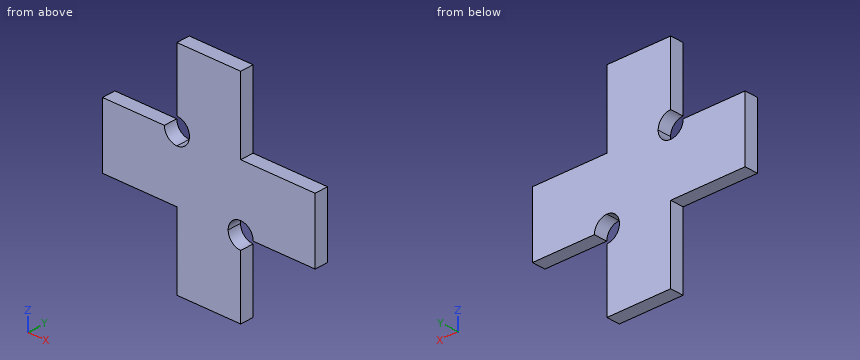
```python
from build123d import *

# Parameters (mm, degrees)
BOSS_EXTRUDE1_DEPTH = 1.6


with BuildPart() as part:
    # Sketch1 → Boss-Extrude1 (new body)
    with BuildSketch(Plane(origin=(0, 0, 0), x_dir=(1, 0, 0), z_dir=(0, 1, 0))):
        with BuildLine():
            Line((-12.7, -3.81), (-5.31, -3.81))
            ThreePointArc((-5.31, -3.81), (-4.870660172, -2.749339828), (-3.81, -2.31))
            Line((-3.81, -2.31), (-3.81, 3.81))
            Line((-3.81, 3.81), (-12.7, 3.81))
            Line((-12.7, 3.81), (-12.7, -3.81))
        make_face()
        with BuildLine():
            Line((-2.31, -3.81), (3.81, -3.81))
            Line((3.81, -3.81), (3.81, 2.31))
            ThreePointArc((3.81, 2.31), (2.749339828, 2.749339828), (2.31, 3.81))
            Line((2.31, 3.81), (-3.81, 3.81))
            Line((-3.81, 3.81), (-3.81, -2.31))
            ThreePointArc((-3.81, -2.31), (-2.749339828, -2.749339828), (-2.31, -3.81))
        make_face()
        with BuildLine():
            Line((-3.81, -12.7), (3.81, -12.7))
            Line((3.81, -12.7), (3.81, -3.81))
            Line((3.81, -3.81), (-2.31, -3.81))
            ThreePointArc((-2.31, -3.81), (-2.749339828, -4.870660172), (-3.81, -5.31))
            Line((-3.81, -5.31), (-3.81, -12.7))
        make_face()
        with BuildLine():
            Line((3.81, 2.31), (3.81, -3.81))
            Line((3.81, -3.81), (12.7, -3.81))
            Line((12.7, -3.81), (12.7, 3.81))
            Line((12.7, 3.81), (5.31, 3.81))
            ThreePointArc((5.31, 3.81), (4.870660172, 2.749339828), (3.81, 2.31))
        make_face()
        with BuildLine():
            Line((-3.81, 3.81), (2.31, 3.81))
            ThreePointArc((2.31, 3.81), (2.749339828, 4.870660172), (3.81, 5.31))
            Line((3.81, 5.31), (3.81, 12.7))
            Line((3.81, 12.7), (-3.81, 12.7))
            Line((-3.81, 12.7), (-3.81, 3.81))
        make_face()
    extrude(amount=BOSS_EXTRUDE1_DEPTH)


solid = part.part
```
Work out the finished part from the listing and answer in its coordinate system (mm). Round coordinates to 2 decimals unless told otherwise and drop trailing zeros. Loops run counter-clockwise (first coordinate to the right, second up) from the corner with the lowest first, then second, coordinate; pieces in that order, holes last.
(1) Each of these flat-tipped pins is pushed along its axis until it touches: P1, Ø0.5, axis at x = -8.5, y = 0.5, coming from the +Z side; P2, Ø0.5, axis at y = 0.5, z = -9.5, coming from the +X side; P3, Ø0.8, axis at x = 10, y = 1, coming from the -Z side; P4, Ø4, axis at x = -6.5, z = 7, coming from the +Y side. Where does it stop, or does it pass through?
Computed values:
P1: stops at z = 3.81
P2: stops at x = 3.81
P3: stops at z = -3.81
P4: passes through
(2) The part is cut by section A-A, the plane x = -3.5. Give the vertices of the cut face in (y, z), and give its area (3 significant figures).
Computed values:
outline: (0, -12.7) - (1.6, -12.7) - (1.6, 2.34) - (0, 2.34) - close; (0, 5.28) - (1.6, 5.28) - (1.6, 12.7) - (0, 12.7) - close
area: 35.9 mm2
(3) The part is cut by section D-D, the plane z = 6.25. Give the vertices of the cut face in (x, y), and give its area (3 significant figures).
Computed values:
outline: (-3.81, 0) - (3.81, 0) - (3.81, 1.6) - (-3.81, 1.6) - close
area: 12.2 mm2
(4) The part is cut by section B-B, the plane y = 1. Give the vertices of the cut face in (x, z).
Computed values:
outline: (-12.7, -3.81) - (-3.81, -3.81) - (-3.81, -12.7) - (3.81, -12.7) - (3.81, -5.31) arc R1.5 cw (long way) to (5.31, -3.81) - (12.7, -3.81) - (12.7, 3.81) - (3.81, 3.81) - (3.81, 12.7) - (-3.81, 12.7) - (-3.81, 5.31) arc R1.5 cw (long way) to (-5.31, 3.81) - (-12.7, 3.81) - close
(5) Find the intervals of material crossed by L1, parallel to Z at x = 3.75, y = 0.65; L2, parallel to X at y = 0.2, z = 11.5, in increasing order.
Computed values:
L1: z = -12.7 to -5.31, -2.31 to 12.7
L2: x = -3.81 to 3.81
(6) The part is cut by section C-C, the plane x = 8.25. Give the vertices of the cut face in (y, z).
Computed values:
outline: (0, -3.81) - (1.6, -3.81) - (1.6, 3.81) - (0, 3.81) - close
